Geometry: see drawing. Coordinates: mm, zero at the bounding-box minimum. Give positions to 0.01 mm unless a question says otherwise; leave off trailing zeros. Use one line per item in the form item = value.
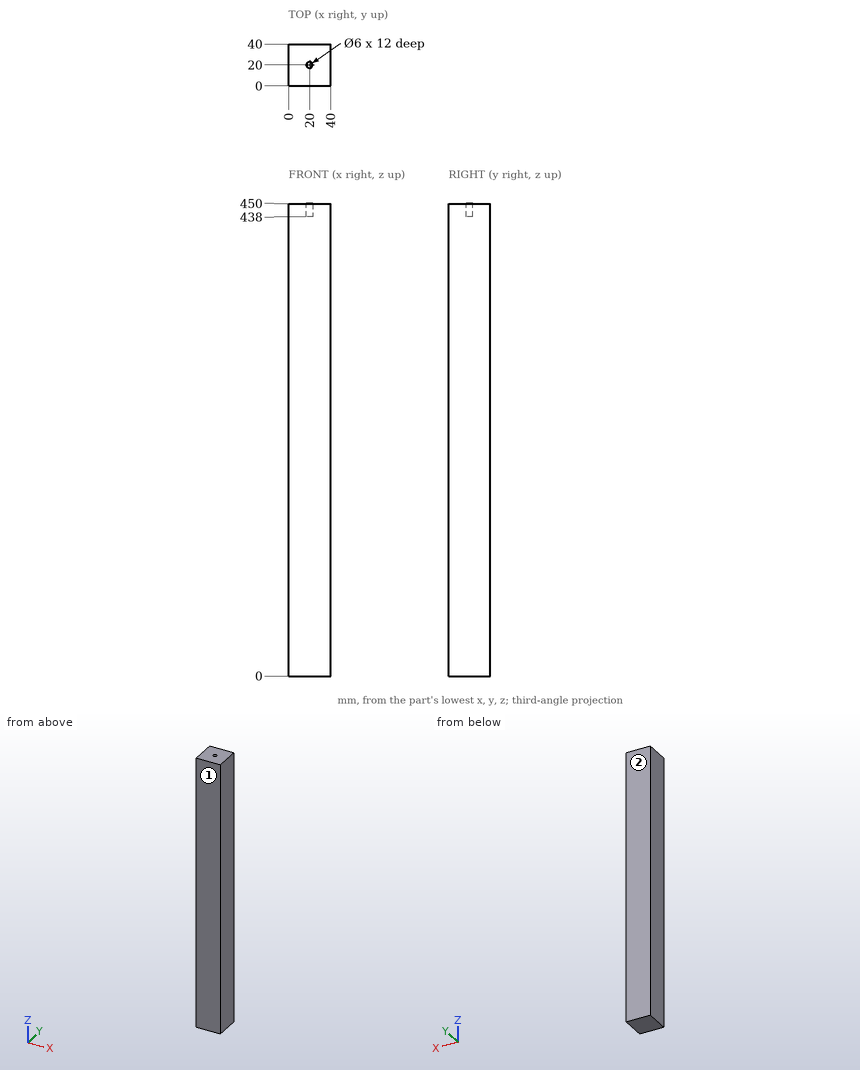
(1) Pin query (flat end, axial travel): P1, Ø5, axis at x = 20, y = 20, coming from the -Z side; P2, Ø1.8, axis at x = 19, y = 20.5, coming from the +Z side. Return the tip coordinate at first contact, or that it passes through.
Solution:
P1 = 0
P2 = 438
(2) Pull-direction query (Y, two-part tool) for the marked faces 1 and 2; classes: released by +Y, released by -Y, zero draft, split by the parting line, or undercut.
Solution:
face_1 = released by -Y
face_2 = released by +Y
(3) Material intervals for L1, parallel to Y at x = 20, z = 445.75, sorted ascending. Write a range as from..to.
Solution:
L1 = 0..17, 23..40
